Source: CAD feature listing. Evaluate the final solid. Frame: model axes, mm. A direction names the side the tool comes from. Round coordinates to 2 decimals unless told otherwise and drop trailing zeros. Loops run counter-clockwise (first coordinate to the right, second up) from the corner with the lowest first, then second, coordinate; pieces in that order, holes last. Notation, with made-up numbers: (21, 3) -> (52, 3) arc R10 ccw to (52, 17) -> close; hole circle Ø8 at (-30.5, 76.25). An arc over 180 degrees is marked (long way). Put each result on its own line as item: value. Start each with the question number.
1. Cut plane C-C (y = 12). Return the cut outline in (x, z).
2. Cut plane A-A (y = -10). Return the cut outline in (x, z), then the cut area to 3 significant figures.
3. Cut plane D-D (x = -29). Return the cut outline in (y, z), then the cut area to 3 significant figures.
4. Material intervals for L1, parallel to Y at x = -16.5, z = -20; L2, parallel to X at y = -18, z = 15; L3, parallel to X at y = 14.5, z = 25, sorted ascending.
5. Contact query for flat-ended pins moving along their axis: pin 1 (1.5 mm diameter, centred on x = -1.5, z = 27, fed in from -Y); pin 2 (3 mm diameter, centred on x = 31, z = 65.5, fed in from +Y); pin 3 (16.5 mm diameter, centred on x = -9.5, z = 12, fed in from +Y). Output: stop coordinate, or through.
6. Set-up query: faces 4 (the flat face through (0, 2, 1)), 5 (the cylindrical face through (-36.125, -19.308, 1.19)), 6 (the flat face through (-36, 0, -85)). Return all of +Z, -Z, +X, -X, +Y, -Y with unobstructed straight access to the full face (end or side cutting, diameter ignored); none if empty.
7. Draft query along X for faces 1 (the flat face through (-40, 0, 1)), 2 (the flat face through (0, -2, 1)), 3 (the flat face through (40, 0, 22)). Return one class per face: pulls with the +X half, pulls with the -X half, needs draft (parallel to the pull), parting line crosses it, or undercut.
8. Cut plane B-B (z = 17). Return the cut outline in (x, y).
```python
from build123d import *

# Parameters (mm, degrees)
VIGA_SB_80_X_6_1_DEPTH     = 170
CORTAR_EXTRUIR1_DEPTH      = 97.046863561
CORTAR_EXTRUIR1_DEPTH_BACK = 97.046863561


with BuildPart() as part:
    # Sketch1 → Viga sb 80 X 6(1) (new body)
    with BuildSketch(Plane.YX.offset(-85)):
        with BuildLine():
            Line((-20, -40), (-20, -38.041460212))
            ThreePointArc((-20, -38.041460212), (-19.289071417, -36.102349063), (-17.493231968, -35.082284275))
            Line((-17.493231968, -35.082284275), (-7.013536064, -33.335540875))
            ThreePointArc((-7.013536064, -33.335540875), (-3.421857166, -31.295411299), (-2, -27.417189001))
            Line((-2, -27.417189001), (-2, 27.417189001))
            ThreePointArc((-2, 27.417189001), (-3.421857166, 31.295411299), (-7.013536064, 33.335540875))
            Line((-7.013536064, 33.335540875), (-17.493231968, 35.082284275))
            ThreePointArc((-17.493231968, 35.082284275), (-19.289071417, 36.102349063), (-20, 38.041460212))
            Line((-20, 38.041460212), (-20, 40))
            Line((-20, 40), (20, 40))
            Line((20, 40), (20, 38.041460212))
            ThreePointArc((20, 38.041460212), (19.289071417, 36.102349063), (17.493231968, 35.082284275))
            Line((17.493231968, 35.082284275), (7.013536064, 33.335540875))
            ThreePointArc((7.013536064, 33.335540875), (3.421857166, 31.295411299), (2, 27.417189001))
            Line((2, 27.417189001), (2, -27.417189001))
            ThreePointArc((2, -27.417189001), (3.421857166, -31.295411299), (7.013536064, -33.335540875))
            Line((7.013536064, -33.335540875), (17.493231968, -35.082284275))
            ThreePointArc((17.493231968, -35.082284275), (19.289071417, -36.102349063), (20, -38.041460212))
            Line((20, -38.041460212), (20, -40))
            Line((20, -40), (-20, -40))
        make_face()
    extrude(amount=VIGA_SB_80_X_6_1_DEPTH)

    # Croquis3 → Cortar-Extruir1 (cut, two sides: drawn at the far end of the back side and taken through both)
    with BuildSketch(Plane(origin=(0, 0, 0), x_dir=(1, 0, 0), z_dir=(0, 1, 0)).offset(-CORTAR_EXTRUIR1_DEPTH_BACK)):
        Polygon((-27.417189001, 85), (71.271160363, 23.404541057), (71.271160363, 105.762435543), (-27.417189001, 105.762435543), align=None)
    extrude(amount=CORTAR_EXTRUIR1_DEPTH + CORTAR_EXTRUIR1_DEPTH_BACK, mode=Mode.SUBTRACT)


solid = part.part
```
Solution:
1. outline: (-40, -85) -> (-34.17, -85) -> (-34.17, 85) -> (-40, 85) -> close; (34.17, -46.56) -> (40, -42.92) -> (40, 85) -> (34.17, 85) -> close
2. outline: (-40, -85) -> (-33.83, -85) -> (-33.83, 85) -> (-40, 85) -> close; (33.83, -46.77) -> (40, -42.92) -> (40, 85) -> (33.83, 85) -> close
2. area: 1,850 mm^2
3. outline: (-2.21, -85) -> (2.21, -85) -> (2.21, 85) -> (-2.21, 85) -> close
3. area: 752 mm^2
4. L1: y = -2 to 2
4. L2: x = -40 to -35.21, 35.21 to 40
4. L3: x = -40 to -34.58, 34.58 to 40
5. pin 1: stops at y = -2
5. pin 2: stops at y = 4.81
5. pin 3: stops at y = 2
6. face 4: +Z, -Z, +Y
6. face 5: +Z, -Z, -Y
6. face 6: -Z, +X, -X, +Y, -Y
7. face 1: pulls with the -X half
7. face 2: undercut
7. face 3: pulls with the +X half
8. outline: (-40, -20) -> (-38.04, -20) arc R3 ccw to (-35.08, -17.49) -> (-33.34, -7.01) arc R6 cw to (-27.42, -2) -> (27.42, -2) arc R6 cw to (33.34, -7.01) -> (35.08, -17.49) arc R3 ccw to (38.04, -20) -> (40, -20) -> (40, 20) -> (38.04, 20) arc R3 ccw to (35.08, 17.49) -> (33.34, 7.01) arc R6 cw to (27.42, 2) -> (-27.42, 2) arc R6 cw to (-33.34, 7.01) -> (-35.08, 17.49) arc R3 ccw to (-38.04, 20) -> (-40, 20) -> close
